```python
from build123d import *

# Parameters (mm, degrees)
BOSS_EXTRUDE1_DEPTH = 1.6
SKETCH2_R           = 1
CUT_EXTRUDE1_DEPTH  = 1.6
SKETCH4_W           = 3.557
SKETCH4_H           = 4.557
BOSS_EXTRUDE2_DEPTH = 0.05


with BuildPart() as part:
    # Sketch1 → Boss-Extrude1 (new body)
    with BuildSketch(Plane(origin=(0, 0, 0), x_dir=(1, 0, 0), z_dir=(0, 1, 0))):
        with BuildLine():
            Line((-10.5, -11.5), (10.5, -11.5))
            ThreePointArc((10.5, -11.5), (11.207106781, -11.207106781), (11.5, -10.5))
            Line((11.5, -10.5), (11.5, 10.5))
            ThreePointArc((11.5, 10.5), (11.207106781, 11.207106781), (10.5, 11.5))
            Line((10.5, 11.5), (-10.5, 11.5))
            ThreePointArc((-10.5, 11.5), (-11.207106781, 11.207106781), (-11.5, 10.5))
            Line((-11.5, 10.5), (-11.5, -10.5))
            ThreePointArc((-11.5, -10.5), (-11.207106781, -11.207106781), (-10.5, -11.5))
        make_face()
    extrude(amount=BOSS_EXTRUDE1_DEPTH)

    # Sketch2 → Cut-Extrude1 (cut)
    with BuildSketch(Plane(origin=(0, 1.6, 0), x_dir=(1, 0, 0), z_dir=(0, 1, 0))):
        with Locations(Location((-8.5, 8.5, 0), (0, 0, 270))):
            Circle(SKETCH2_R)
        with Locations(Location((-8.5, -8.5, 0), (0, 0, 90))):
            Circle(SKETCH2_R)
        with Locations(Location((8.5, 8.5, 0), (0, 0, 90))):
            Circle(SKETCH2_R)
        with Locations(Location((8.5, -8.5, 0), (0, 0, 270))):
            Circle(SKETCH2_R)
    extrude(amount=-CUT_EXTRUDE1_DEPTH, mode=Mode.SUBTRACT)

    # Sketch4 → Boss-Extrude2 (add)
    with BuildSketch(Plane(origin=(0, 1.6, 0), x_dir=(1, 0, 0), z_dir=(0, 1, 0))):
        Rectangle(SKETCH4_W, SKETCH4_H)
    extrude(amount=BOSS_EXTRUDE2_DEPTH)


solid = part.part
```
Source: CAD feature listing. Evaluate the final solid. Frame: model axes, mm. Round coordinates to 2 decimals unless told otherwise and drop trailing zeros. Write each loop counter-clockwise with the first axis right and the second up, starting at its lowest first coordinate (ties: lowest second). Pieces come first, ordered by that corner, then holes. Notation, with made-up numbers: M 67,2 L 100,2 A35 ccw 100,34 Z; hole C 55.5,24 d10. An arc over 180 degrees is marked long. Answer as a JSON object with one key per item and string values. Group by question number.
(1) Mould query, pull axis Z, two halves, no side actions, for faces 1 (the cylindrical face through (9.49, 0.81, 8.37)), 2 (the cylindrical face through (-11.199, 0.789, -11.215)), 3 (the flat face through (0, 1, 11.5)). Classes: +Z half, -Z half, draft (parallel to the pull), parting line (faces both ways), or undercut.
(2) Section query C-C on y = 0.55. Output: boundary loops of the cut face in (x, z), then the cut area to 3 significant figures.
(3) Section query B-B on z = -8.5. Output: boundary loops of the cut face in (x, y).
(4) Ray query, line 1 (X direction, y = 0.7, z = -8.5); line 2 (Y direction, x = -6, z = 0). Return the intervals inside material, ascending. Write a range as [from, to].
(5) First-contact query: pin 1 (1.5 mm diameter, centred on x = 8.5, z = 5.5, fed in from -Y); pin 2 (2.5 mm diameter, centred on x = -8.5, z = 8.5, fed in from +Y); pin 3 (1.2 mm diameter, centred on x = 8.5, z = -8.5, fed in from +Y). Flat tips, straight axial feed; report the tip coordinate or a pass-through.
(6) Section query D-D on z = -1.25. Output: boundary loops of the cut face in (x, y), then the cut area to 3 significant figures.
(7) Section query A-A on x = 8.5. Output: boundary loops of the cut face in (y, z), then the cut area to 3 significant figures.
Computed values:
{
 "1": {"face 1": "undercut", "face 2": "-Z half", "face 3": "+Z half"},
 "2": {"outline": "M -11.5,-10.5 A1 ccw -10.5,-11.5 L 10.5,-11.5 A1 ccw 11.5,-10.5 L 11.5,10.5 A1 ccw 10.5,11.5 L -10.5,11.5 A1 ccw -11.5,10.5 Z; hole C -8.5,-8.5 d2; hole C -8.5,8.5 d2; hole C 8.5,-8.5 d2; hole C 8.5,8.5 d2", "area": "516 mm^2"},
 "3": {"outline": "M -11.5,0 L -9.5,0 L -9.5,1.6 L -11.5,1.6 Z; M -7.5,0 L 7.5,0 L 7.5,1.6 L -7.5,1.6 Z; M 9.5,0 L 11.5,0 L 11.5,1.6 L 9.5,1.6 Z"},
 "4": {"line 1": "[-11.5, -9.5], [-7.5, 7.5], [9.5, 11.5]", "line 2": "[0, 1.6]"},
 "5": {"pin 1": "y = 0", "pin 2": "y = 1.6", "pin 3": "through"},
 "6": {"outline": "M -11.5,0 L 11.5,0 L 11.5,1.6 L 1.78,1.6 L 1.78,1.65 L -1.78,1.65 L -1.78,1.6 L -11.5,1.6 Z", "area": "37.0 mm^2"},
 "7": {"outline": "M 0,-11.5 L 1.6,-11.5 L 1.6,-9.5 L 0,-9.5 Z; M 0,-7.5 L 1.6,-7.5 L 1.6,7.5 L 0,7.5 Z; M 0,9.5 L 1.6,9.5 L 1.6,11.5 L 0,11.5 Z", "area": "30.4 mm^2"}
}
